Verification items for this drawing (mm, ordinates from the low corner). A direction names the side the tool comes from. Give positions to 0.01 mm unless a question says otherwise; leave off trailing zeros. Write each loop counter-clockwise with the first axis right and the second up, starting at its lowest first coordinate (ties: lowest second). Pieces come first, ordered by that corner, then holes. Notation, with made-up numbers: (80.25, -29.5) -> (118.25, -29.5) arc R9 cw to (118.25, -22.5) -> close; hole circle Ø6 at (18, -39). An arc over 180 degrees is marked (long way). Answer as a JSON object with one key per item and string values.
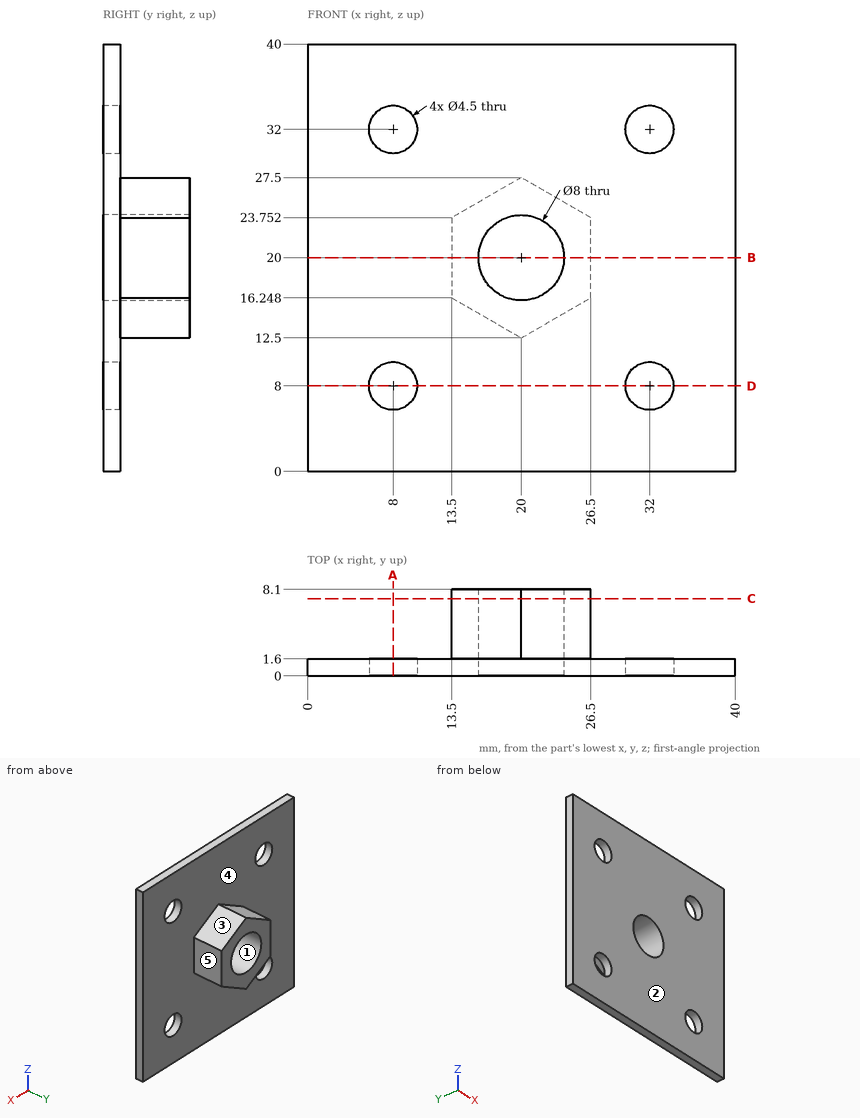
1. Sectioned sample at B-B, the plane z = 20. Enter the section's corners in (x, y).
Determined:
{"outline": "(0, 0) -> (16, 0) -> (16, 8.1) -> (13.5, 8.1) -> (13.5, 1.6) -> (0, 1.6) -> close; (24, 0) -> (40, 0) -> (40, 1.6) -> (26.5, 1.6) -> (26.5, 8.1) -> (24, 8.1) -> close"}
2. Go/stop test with flat-tipped pins: P1, Ø3, axis at y = 5.5, z = 20.5, coming from the -X side; P2, Ø5, axis at x = 32, z = 8, coming from the +Y side. Record where each tip stops, or that it passes through.
Determined:
{"P1": "x = 13.5", "P2": "y = 1.6"}
3. Sectioned sample at A-A, the plane x = 8. Enter the section's corners in (y, z).
Determined:
{"outline": "(0, 0) -> (1.6, 0) -> (1.6, 5.75) -> (0, 5.75) -> close; (0, 10.25) -> (1.6, 10.25) -> (1.6, 29.75) -> (0, 29.75) -> close; (0, 34.25) -> (1.6, 34.25) -> (1.6, 40) -> (0, 40) -> close"}
4. Sectioned sample at C-C, the plane y = 7.25. Enter the section's corners in (x, z).
Determined:
{"outline": "(13.5, 16.25) -> (20, 12.5) -> (26.5, 16.25) -> (26.5, 23.75) -> (20, 27.5) -> (13.5, 23.75) -> close; hole circle Ø8 at (20, 20)"}
5. Scan lines: L1, parallel to X at y = 1.2, z = 8; L2, parallel to X at y = 5, z = 20; L3, parallel to Y at x = 6, z = 34. Record each from-to range of solid material in increasing order. Write a range as [from, to].
Determined:
{"L1": "[0, 5.75], [10.25, 29.75], [34.25, 40]", "L2": "[13.5, 16], [24, 26.5]", "L3": "[0, 1.6]"}
6. Mould release check, pull along X, two halves, no side actions. Record for the marked faces 1, 2 and 3: released by +X, released by -X, zero draft, split by the parting line, or undercut.
Determined:
{"face 1": "undercut", "face 2": "zero draft", "face 3": "released by +X"}
7. Access from +Z, -Z, +X, -X, +Y, -Y to the whole of each face (thin tool, end or side, straight path). Record for the marked faces 4 and 5.
Determined:
{"face 4": "+Y", "face 5": "+Z, -Z, +X, +Y"}
8. Sectioned sample at D-D, the plane z = 8. Enter the section's corners in (x, y).
Determined:
{"outline": "(0, 0) -> (5.75, 0) -> (5.75, 1.6) -> (0, 1.6) -> close; (10.25, 0) -> (29.75, 0) -> (29.75, 1.6) -> (10.25, 1.6) -> close; (34.25, 0) -> (40, 0) -> (40, 1.6) -> (34.25, 1.6) -> close"}
